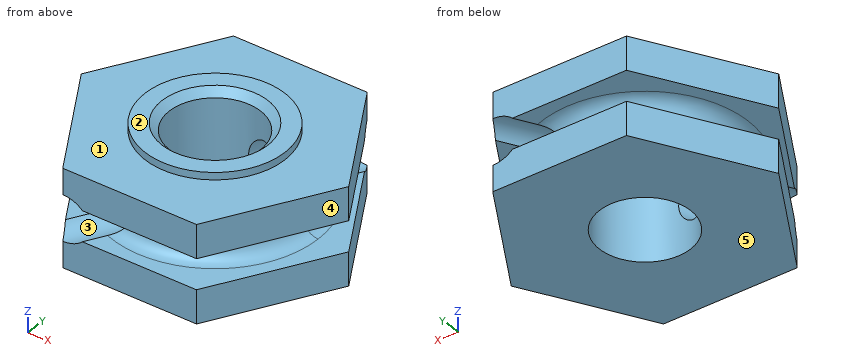
```python
from build123d import *

# Parameters (mm, degrees)
BOSS_EXTRUDE1_DEPTH = 2.54
SKETCH2_R           = 3.65125
SKETCH2_R_2         = 2.38125
BOSS_EXTRUDE2_DEPTH = 0.381
SKETCH3_R           = 2.38125
CUT_EXTRUDE1_DEPTH  = 11.522303198
CHAMFER1_SIZE       = 0.381
SKETCH4_R           = 1.19126
CUT_EXTRUDE2_DEPTH  = 17.225585806


with BuildPart() as part:
    # Sketch1 → Boss-Extrude1 (new, symmetric)
    with BuildSketch(Plane.XY):
        Polygon((3.482865499, 6.0325), (-3.482865499, 6.0325), (-6.965730998, 0), (-3.482865499, -6.0325), (3.482865499, -6.0325), (6.965730998, 0), align=None)
    extrude(amount=BOSS_EXTRUDE1_DEPTH, both=True)

    # Sketch2 → Boss-Extrude2 (add)
    with BuildSketch(Plane.XY.offset(2.54)):
        with Locations(Location((0, 0, 0), (0, 0, 180))):
            Circle(SKETCH2_R)
        with Locations(Location((0, 0, 0), (0, 0, 180))):
            Circle(SKETCH2_R_2, mode=Mode.SUBTRACT)
    extrude(amount=BOSS_EXTRUDE2_DEPTH)

    # Sketch3 → Cut-Extrude1 (cut, through all)
    with BuildSketch(Plane.XY.offset(2.54)):
        with Locations(Location((0, 0, 0), (0, 0, 180))):
            Circle(SKETCH3_R)
    extrude(amount=-CUT_EXTRUDE1_DEPTH, mode=Mode.SUBTRACT)

    # Chamfer1
    chamfer1_edges = [part.edges().sort_by_distance(p)[0] for p in [
        (2.38125, 0, 2.921),
    ]]
    chamfer(chamfer1_edges, length=CHAMFER1_SIZE - 0.0001)  # a hair under: the kernel refuses the full size

    # Sketch4 → Cut-Extrude2 (cut, through all)
    with BuildSketch(Plane(origin=(3.482865499, 6.0325, 0), x_dir=(0, 0, -1), z_dir=(-0.49999999999999944, -0.8660254037844389, 0))):
        with Locations(Location((0, 0, 0), (0, 0, 270))):
            Circle(SKETCH4_R)
    extrude(amount=CUT_EXTRUDE2_DEPTH, mode=Mode.SUBTRACT)

    # Sketch5 → Cut-Revolve1 (revolve, cut)
    with BuildSketch(Plane(origin=(0, 0, 0), x_dir=(0, 0, 1), z_dir=(-0.8660254037844389, 0.4999999999999995, 0)), mode=Mode.PRIVATE) as cut_revolve1_sk:
        with BuildLine():
            Line((-0.79375, 6.965730998), (-0.79375, 5.378230998))
            ThreePointArc((-0.79375, 5.378230998), (0, 4.584480998), (0.79375, 5.378230998))
            Line((0.79375, 5.378230998), (0.79375, 6.965730998))
            Line((0.79375, 6.965730998), (-0.79375, 6.965730998))
        make_face()
    revolve(cut_revolve1_sk.sketch.rotate(Axis((0, 0, -1000.088934232), (0, 0, 1)), 300), axis=Axis((0, 0, -1000.088934232), (0, 0, 1)), mode=Mode.SUBTRACT)


solid = part.part
```
Read the model definition and answer for the solid it produces. Units are mm, in the model's axes. Face numbers are marked on the shaded views. A direction names the side the tool comes from. Give positions to 0.01 mm unless a question says otherwise; leave off trailing zeros. Loops run counter-clockwise (first coordinate to the right, second up) from the corner with the lowest first, then second, coordinate; pieces in that order, holes last.
Item 1: Each of these flat-tipped pins is pushed along its axis until it touches: pin 1 Ø4 at (x, y) = (0, 0) entering from -Z; pin 2 Ø1.5 at (y, z) = (-3, 1.5) entering from +X; pin 3 Ø1.5 at (x, z) = (5.5, -1.5) entering from +Y. Where does it stop, or does it pass through?
Item 2: Find the intervals of material crossed by line 1 along Y through (x, z) = (0, 2.5); line 2 along Z through (x, y) = (5.25, -2); line 3 along Z through (x, y) = (3.25, 5.5), in increasing order.
Item 3: The mould has two halves that part along X. Classify the marked faces 3, 4 and 5: released by +X, released by -X, zero draft, split by the parting line, or undercut.
Item 4: For the marked faces 1 and 2, determine the directions among +Z, -Z, +X, -X, +Y, -Y from which every point of the face is accessible in a straight line to the end or side of a thin tool.
Item 5: The part is cut by section A-A (z = -0.35). Write down the section's boundary in (x, y).
Taken from the geometry:
1. pin 1: passes through
1. pin 2: stops at x = 5.67
1. pin 3: stops at y = 3.84
2. line 1: y = -6.03 to -2.38, 2.38 to 6.03
2. line 2: z = -2.54 to -0.79, 0.79 to 2.54
2. line 3: z = -2.54 to -1.19, 1.19 to 2.54
3. face 3: undercut
3. face 4: released by +X
3. face 5: zero draft
4. face 1: +Z
4. face 2: +Z, +X, -X, +Y, -Y
5. outline: (-3.25, -3.35) - (-2.03, -1.24) arc R2.38 cw to (0.06, 2.38) - (1.28, 4.49) arc R4.67 ccw to start; (-1.28, -4.49) arc R4.67 ccw to (3.25, 3.35) - (2.03, 1.24) arc R2.38 cw to (-0.06, -2.38) - close
